The listing builds one solid part. Answer for the finished solid, in the listing's coordinates (mm). Give positions to 0.01 mm unless a question says otherwise; leave off trailing zeros. Write each loop counter-clockwise with the first axis right and the second up, starting at its lowest first coordinate (ties: lowest second). Pieces come first, ordered by that corner, then holes. Notation, with made-up numbers: (52.25, 25.5) - (72.25, 25.5) arc R13 ccw to (72.25, 41.5) - close; hole circle Ø6 at (64, 46.25). An arc over 180 degrees is marked (long way). Answer as CSV lines item,"result". Start each with the question number.
(1) This flat-tipped pin is pushed along its axis until it touches: pin 1 Ø4 at (x, y) = (66.02, -133.01) entering from +Z. Where does it stop, or does it pass through?
(2) Straight lines are drawn through the part: probe 1 along X at (y, z) = (-83, 11.2); probe 2 along X at (y, z) = (-95.5, 9.4); probe 3 along Y at (x, z) = (82.5, 10.25). For each, find the intervals that lie inside material, in ascending order.
(3) Find section A-A (y = -122.65). Write down the section's boundary in (x, z), then the cut area to 3 significant figures.
(4) Find section C-C (x = 71). Write down the section's boundary in (y, z).
(5) Find section D-D (z = 9.7). State how many separate pieces and enclosed holes the cut face has, then the cut area to 3 significant figures.
(6) For a pull along X with two mould halves and no side action, classify faces 1 (the face through (148.713, -39.273, 10.178)), 2 (the face through (92, -85, 11.43)), 3 (the face through (66.696, -134.316, 10.178)) as pulls with the +X half, pulls with the -X half, needs draft (parallel to the pull), parting line crosses it, or undercut.
(7) Find section B-B (x = 116). Write down the section's boundary in (y, z), then the cut area to 3 significant figures.
from build123d import *

# Parameters (mm, degrees)
SKETCH2_W           = 116.725527873
SKETCH2_H           = 133.165089742
BOSS_EXTRUDE1_DEPTH = 2.54
SKETCH3_W           = 20.623543236
SKETCH3_H           = 21.169862262
SKETCH3_W_2         = 20.760122992
SKETCH3_H_2         = 20.48696348
SKETCH3_W_3         = 21.306442018
SKETCH3_H_3         = 19.940644453
CUT_EXTRUDE1_DEPTH  = 2.54
SKETCH5_R           = 7.656955564
CUT_EXTRUDE3_DEPTH  = 2.54
SKETCH7_W           = 11.00850593
SKETCH7_H           = 30.296913756
CUT_EXTRUDE4_DEPTH  = 2.54
SKETCH8_R           = 1.475
CUT_EXTRUDE6_DEPTH  = 2.95


with BuildPart() as part:
    # Sketch2 → Boss-Extrude1 (new body)
    with BuildSketch(Plane.XY.offset(8.89)):
        with Locations((105.793885205, -85.85721005)):
            Rectangle(SKETCH2_W, SKETCH2_H)
    extrude(amount=BOSS_EXTRUDE1_DEPTH)

    # Sketch3 → Cut-Extrude1 (cut)
    with BuildSketch(Plane.XY.offset(11.43)):
        with Locations((76.576493833, -105.769912046)):
            Rectangle(SKETCH3_W, SKETCH3_H)
        with Locations((110.51656333, -84.941499175)):
            Rectangle(SKETCH3_W_2, SKETCH3_H_2)
        with Locations((76.917943224, -66.503232044)):
            Rectangle(SKETCH3_W_3, SKETCH3_H_3)
    extrude(amount=-CUT_EXTRUDE1_DEPTH, mode=Mode.SUBTRACT)

    # Sketch5 → Cut-Extrude3 (cut)
    with BuildSketch(Plane.XY.offset(11.43)):
        with Locations((135.8, -122.65)):
            Circle(SKETCH5_R)
    extrude(amount=-CUT_EXTRUDE3_DEPTH, mode=Mode.SUBTRACT)

    # Sketch7 → Cut-Extrude4 (cut)
    with BuildSketch(Plane.XY.offset(11.43)):
        with Locations((136.149279083, -84.937713867)):
            Rectangle(SKETCH7_W, SKETCH7_H)
    extrude(amount=-CUT_EXTRUDE4_DEPTH, mode=Mode.SUBTRACT)

    # Sketch8 → Cut-Extrude6 (cut)
    with BuildSketch(Plane.XY.offset(11.43)):
        with Locations((66.015339877, -133.007279185)):
            Circle(SKETCH8_R)
        with Locations((148.032128518, -37.964511979)):
            Circle(SKETCH8_R)
    extrude(amount=-CUT_EXTRUDE6_DEPTH, mode=Mode.SUBTRACT)


solid = part.part
Result set:
1,pin 1,"z = 11.43"
2,probe 1,"47.43 to 100.14, 120.9 to 130.65, 141.65 to 164.16"
2,probe 2,"47.43 to 66.26, 86.89 to 130.65, 141.65 to 164.16"
2,probe 3,"-152.44 to -116.35, -95.18 to -76.47, -56.53 to -19.27"
3,outline,"(47.43, 8.89) - (128.14, 8.89) - (128.14, 11.43) - (47.43, 11.43) - close; (143.46, 8.89) - (164.16, 8.89) - (164.16, 11.43) - (143.46, 11.43) - close"
3,area,"258 mm^2"
4,outline,"(-152.44, 8.89) - (-116.35, 8.89) - (-116.35, 11.43) - (-152.44, 11.43) - close; (-95.18, 8.89) - (-76.47, 8.89) - (-76.47, 11.43) - (-95.18, 11.43) - close; (-56.53, 8.89) - (-19.27, 8.89) - (-19.27, 11.43) - (-56.53, 11.43) - close"
5,separate pieces,"1"
5,enclosed holes,"7"
5,area,"13,700 mm^2"
6,face 1,"undercut"
6,face 2,"needs draft"
6,face 3,"undercut"
7,outline,"(-152.44, 8.89) - (-95.18, 8.89) - (-95.18, 11.43) - (-152.44, 11.43) - close; (-74.7, 8.89) - (-19.27, 8.89) - (-19.27, 11.43) - (-74.7, 11.43) - close"
7,area,"286 mm^2"
